from build123d import *

# Parameters (mm, degrees)
F0_W      = 29
F0_H      = 16.5
F1_DEPTH  = 38.5
F2_T      = -2
F3_DEPTH  = 2.25
F4_SIZE   = 2
F5_SIZE   = 2
F6_SIZE   = 1
F8_DEPTH  = 16.501
F10_DEPTH = 2
F11_R     = 2
F12_DEPTH = 2.001
F13_W     = 7.54
F13_H     = 7.25
F13_R     = 1.1
F14_DEPTH = 4.35


with BuildPart() as f1:
    # F0 (on Top) → F1 (new body)
    with BuildSketch(Plane.XY):
        with Locations((14.5, 8.25)):
            Rectangle(F0_W, F0_H)
    extrude(amount=F1_DEPTH)

    # F2
    f2_openings = [f1.faces().sort_by_distance(p)[0] for p in [
        (14.5, 8.25, 38.5),
    ]]
    offset(amount=F2_T, openings=f2_openings)

    # F3 (add): a face of the model
    f3_faces = [f1.faces().sort_by_distance(p)[0] for p in [
        (14.5, 8.25, 2),
    ]]
    extrude(f3_faces, amount=F3_DEPTH)

    # F4
    f4_edges = [f1.edges().sort_by_distance(p)[0] for p in [
        (29, 0, 19.25),
        (29, 16.5, 19.25),
        (0, 16.5, 19.25),
        (0, 0, 19.25),
    ]]
    chamfer(f4_edges, length=F4_SIZE)

    # F5 (call 1 of 4: OpenCascade refuses the feature's edges together)
    f5_edges = [f1.edges().sort_by_distance(p)[0] for p in [
        (14.5, 0, 0),
    ]]
    chamfer(f5_edges, length=F5_SIZE)

    # F5#2 (call 2 of 4)
    f5_2_edges = [f1.edges().sort_by_distance(p)[0] for p in [
        (29, 8.25, 0),
    ]]
    chamfer(f5_2_edges, length=F5_SIZE)

    # F5#3 (call 3 of 4)
    f5_3_edges = [f1.edges().sort_by_distance(p)[0] for p in [
        (0, 8.25, 0),
    ]]
    chamfer(f5_3_edges, length=F5_SIZE)

    # F5#4 (call 4 of 4)
    f5_4_edges = [f1.edges().sort_by_distance(p)[0] for p in [
        (14.5, 16.5, 0),
    ]]
    chamfer(f5_4_edges, length=F5_SIZE)

    # F6
    f6_edges = [f1.edges().sort_by_distance(p)[0] for p in [
        (29, 8.25, 38.5),
        (28, 15.5, 38.5),
        (14.5, 16.5, 38.5),
        (1, 15.5, 38.5),
        (0, 8.25, 38.5),
        (1, 1, 38.5),
        (14.5, 0, 38.5),
        (28, 1, 38.5),
    ]]
    chamfer(f6_edges, length=F6_SIZE)

    # F7 (on face) → F8 (cut, through all)
    with BuildSketch(Plane.XZ):
        Polygon((6.464, 8.664), (6.464, 4.94), (23.536, 4.94), (23.536, 8.664), (17.364, 12.834), (12.635, 12.834), align=None)
    extrude(amount=-F8_DEPTH, mode=Mode.SUBTRACT)

    # F9 (on face) → F10 (cut, through all)
    with BuildSketch(Plane.YZ.offset(29)):
        with BuildLine():
            ThreePointArc((5.0038961688, 23.1590909091), (8.1704306945, 19.7509741882), (11.5, 23))
            ThreePointArc((11.5, 23), (11.4990258118, 23.0795693055), (11.4961038312, 23.1590909091))
            ThreePointArc((11.4961038312, 23.1590909091), (8.25, 22.25), (5.0038961688, 23.1590909091))
        make_face()
        with BuildLine():
            ThreePointArc((5.0038961688, 23.1590909091), (8.25, 22.25), (11.4961038312, 23.1590909091))
            ThreePointArc((11.4961038312, 23.1590909091), (8.25, 26.25), (5.0038961688, 23.1590909091))
        make_face()
        with BuildLine():
            ThreePointArc((5.0038961688, 23.1590909091), (8.25, 26.25), (11.4961038312, 23.1590909091))
            ThreePointArc((11.4961038312, 23.1590909091), (13.6975062618, 25.4361502113), (14.5, 28.5))
            Line((14.5, 28.5), (2, 28.5))
            ThreePointArc((2, 28.5), (2.8024937382, 25.4361502113), (5.0038961688, 23.1590909091))
        make_face()
        with BuildLine():
            Line((2, 28.5), (14.5, 28.5))
            ThreePointArc((14.5, 28.5), (8.25, 34.75), (2, 28.5))
        make_face()
        with BuildLine():
            ThreePointArc((2, 28.5), (8.25, 34.75), (14.5, 28.5))
            Line((14.5, 28.5), (14.5, 38.5))
            Line((14.5, 38.5), (2, 38.5))
            Line((2, 38.5), (2, 28.5))
        make_face()
    extrude(amount=-F10_DEPTH, mode=Mode.SUBTRACT)

    # F11 (on face) → F12 (cut, through all)
    with BuildSketch(Plane.YZ.offset(2)):
        with Locations((8.25, 23)):
            Circle(F11_R)
    extrude(amount=-F12_DEPTH, mode=Mode.SUBTRACT)

    # F13 (on face) → F14 (join)
    with BuildSketch(Plane.YZ.offset(2)):
        with Locations((8.25, 7.875)):
            Rectangle(F13_W, F13_H)
        with Locations((8.25, 9)):
            Circle(F13_R, mode=Mode.SUBTRACT)
    extrude(amount=F14_DEPTH)


solid = f1.part
Could you check a few things on this model? Use its own coordinates, in mm. A direction names the side the tool comes from. Give positions to 0.01 mm unless a question says otherwise; leave off trailing zeros. Order: outer loops, then holes, each group sorted by start corner. A loop starts at its lowest first (then second) coordinate and runs counter-clockwise, first axis right, second up. Notation, with made-up numbers: (-14, -12.75) - (19, -12.75) arc R18 cw to (19, -5.75) - close; hole circle Ø8 at (9, -20.5). An arc over 180 degrees is marked (long way). One line per item, written item: value. Start each with the question number.
1. Imagine slicing it at D-D on x = 24.5. List the corners of the cut face in (y, z) for me, plus the area to 3 significant figures.
2. Imagine slicing it at C-C on z = 15. List the corners of the cut face in (x, y) for me.
3. For P1, Ø0.6, axis at y = 1, z = 7, coming from the +X side; P2, Ø3, axis at x = 11.5, z = 6.5, coming from the +Y side, each with a flat end and sliding along its axis, tell me the tip position at first contact or that it passes through.
4. If I drill on probe 1 along X at (y, z) = (3.75, 16); probe 2 along Y at (x, z) = (14.5, 28.5); probe 3 along X at (y, z) = (5.25, 4.5), over which ranges is the centre line in solid material (lowest first)?
5. For faces 1 (the face through (28.01, 2.78, 25.48)), 2 (the face through (27.706, 1.266, 37.896)), 3 (the face through (27, 8, 14)), 4 (the face through (9.593, 0.986, 10.778)), 5 (the face through (14, 1, 1)), which set-ups out of +Z, -Z, +X, -X, +Y, -Y let a thin tool reach every point of the face, with its end or its side?
6. Thinking about a two-plate mould opening in Z: for faces 6 (the face through (12, 15, 38.5)), 7 (the face through (15, 1, 4.94)), 8 (the face through (4, 12.02, 8)), which applies, +Z half, -Z half, draft (parallel to the pull), parting line (faces both ways), or undercut?
7. Imagine slicing it at A-A on x = 14.75. List the corners of the cut face in (y, z) for me, plus the area to 3 significant figures.
8. Imagine slicing it at B-B on y = 8.25. List the corners of the cut face in (x, z) for me.
Values:
1. outline: (0, 2) - (2, 0) - (14.5, 0) - (16.5, 2) - (16.5, 37.5) - (15.5, 38.5) - (14.5, 38.5) - (14.5, 4.25) - (2, 4.25) - (2, 38.5) - (1, 38.5) - (0, 37.5) - close
1. area: 202 mm²
2. outline: (0, 2) - (2, 0) - (27, 0) - (29, 2) - (29, 14.5) - (27, 16.5) - (2, 16.5) - (0, 14.5) - close; hole (2, 2) - (27, 2) - (27, 14.5) - (2, 14.5) - close
3. P1: x = 28.3
3. P2: through
4. probe 1: 0 to 2, 27 to 29
4. probe 2: 0 to 2, 14.5 to 16.5
4. probe 3: 0 to 6.35, 27 to 29
5. face 1: +Z, +X
5. face 2: +Z, +X, -Y
5. face 3: +Z
5. face 4: +Y, -Y
5. face 5: -Z, +X, -X, -Y
6. face 6: +Z half
6. face 7: undercut
6. face 8: draft
7. outline: (0, 2) - (2, 0) - (14.5, 0) - (16.5, 2) - (16.5, 4.94) - (14.5, 4.94) - (14.5, 4.25) - (2, 4.25) - (2, 4.94) - (0, 4.94) - close; (0, 12.83) - (2, 12.83) - (2, 38.5) - (1, 38.5) - (0, 37.5) - close; (14.5, 12.83) - (16.5, 12.83) - (16.5, 37.5) - (15.5, 38.5) - (14.5, 38.5) - close
7. area: 171 mm²
8. outline: (0, 2) - (2, 0) - (27, 0) - (29, 2) - (29, 19.75) - (27, 19.75) - (27, 4.25) - (6.35, 4.25) - (6.35, 7.9) - (2, 7.9) - (2, 10.1) - (6.35, 10.1) - (6.35, 11.5) - (2, 11.5) - (2, 21) - (0, 21) - close; (0, 25) - (2, 25) - (2, 38.5) - (1, 38.5) - (0, 37.5) - close
